Autodesk Inventor part; units mm, degrees
ref_plane "YZ Plane" through (0, 0, 0) normal (1, 0, 0) x (0, 1, 0)
ref_plane "XZ Plane" through (0, 0, 0) normal (0, 1, 0) x (-1, 0, 0)
ref_plane "XY Plane" through (0, 0, 0) normal (0, 0, 1) x (1, 0, 0)
sketch "Sketch1" plane through (0, 0, 0) normal (0, 1, 0) x (-1, 0, 0)
  line L0 (0, 0) -> (-215.9, 0)
  line L1 (-215.9, 0) -> (-215.9, -132.08)
  line L2 (-215.9, -132.08) -> (0, -132.08)
  line L3 (0, -132.08) -> (0, 0)
  circle A0 centre (-46.99, -129.008) radius 1.65
  circle A1 centre (-168.91, -129.008) radius 1.65
  circle A2 centre (-46.99, -3.072) radius 1.65
  circle A3 centre (-168.91, -3.072) radius 1.65
  circle A4 centre (-8, -50) radius 2.2
  circle A5 centre (-8, -100) radius 2.2
  circle A6 centre (-58, -50) radius 2.2
  circle A7 centre (-58, -100) radius 2.2
  circle A8 centre (-108, -50) radius 2.2
  circle A9 centre (-108, -100) radius 2.2
  circle A10 centre (-158, -50) radius 2.2
  circle A11 centre (-158, -100) radius 2.2
  circle A12 centre (-52.45, -72.08) radius 1.25
  circle A13 centre (-163.45, -72.08) radius 1.25
  circle A14 centre (-52.45, -33.08) radius 1.25
  circle A15 centre (-163.45, -33.08) radius 1.25
  dimension "d0" = 215.9
  dimension "d1" = 132.08
  dimension "d2" = 3.3
  dimension "d5" = 121.92
  dimension "d8" = 125.936
  dimension "d11" = 46.99
  dimension "d12" = 3.072
  dimension "d13" = 3.072
  dimension "d14" = 4.4
  dimension "d15" = 50
  dimension "d16" = 8
  dimension "d19" = 50
  dimension "d22" = 50
  dimension "d30" = 2.5
  dimension "d33" = 111
  dimension "d36" = 39
  dimension "d39" = 60
  dimension "d40" = 52.45
extrude "Extrusion1" add sketch "Sketch1" against normal blind 2.54
sketch "Sketch2" plane through (0, 0, 0) normal (0, 1, 0) x (1, 0, 0)
  line L0 (108.9107, 44.2653) -> (116.6369, 44.2653) construction
  line L1 (116.6369, 44.2653) -> (116.6369, 41.0888) construction
  line L2 (116.6369, 41.0888) -> (108.9107, 41.0888) construction
  line L3 (108.9107, 41.0888) -> (108.9107, 44.2653) construction
  point P0 (0, 0)
extrude "Extrusion2" [suppressed]
fillet "Fillet1" radius 5 4 edges at (0, -1.27, 0) (215.9, -1.27, 0) (215.9, -1.27, -132.08) (0, -1.27, -132.08)
sketch "Sketch3" plane through (0, 0, 0) normal (0, 1, 0) x (1, 0, 0)
  arc A0 (5, 132.08) -> (0, 127.08) centre (5, 127.08) ccw
  line L0 (0, 127.08) -> (0, 5)
  arc A1 (0, 5) -> (5, 0) centre (5, 5) ccw
  line L1 (5, 0) -> (210.9, 0)
  arc A2 (210.9, 0) -> (215.9, 5) centre (210.9, 5) ccw
  line L2 (215.9, 5) -> (215.9, 127.08)
  arc A3 (215.9, 127.08) -> (210.9, 132.08) centre (210.9, 127.08) ccw
  line L3 (210.9, 132.08) -> (5, 132.08)
  circle A4 centre (163.45, 33.08) radius 1.25
  circle A5 centre (163.45, 72.08) radius 1.25
  circle A6 centre (158, 100) radius 2.2
  circle A7 centre (108, 100) radius 2.2
  circle A8 centre (58, 100) radius 2.2
  circle A9 centre (58, 50) radius 2.2
  circle A10 centre (8, 100) radius 2.2
  circle A11 centre (8, 50) radius 2.2
  circle A12 centre (168.91, 3.072) radius 1.65
  circle A13 centre (46.99, 3.072) radius 1.65
  circle A14 centre (168.91, 129.008) radius 1.65
  circle A15 centre (46.99, 129.008) radius 1.65
  circle A16 centre (108, 50) radius 2.2
  circle A17 centre (158, 50) radius 2.2
  circle A18 centre (52.45, 72.08) radius 1.25
  circle A19 centre (52.45, 33.08) radius 1.25
  point P0 (0, 0)
equation "\"d40\" = -0.5 * d33 + 0.5 * d0"
properties part number "amplifier_tray"
Geometry check sheet. Reference: the model listing, model coordinates, mm. Round coordinates to 2 decimals unless told otherwise and drop trailing zeros. Order: outer loops, then holes, each group sorted by start corner. A loop starts at its lowest first (then second) coordinate and runs counter-clockwise, first axis right, second up. Notation, with made-up numbers: M 21,-38 L 68,-38 A26 ccw 68,-7 Z; hole C 49.5,-17.75 d11. An arc over 180 degrees is marked long. Answer as CSV lines item,"result".
1) Sectioned sample at A-A on x = 8. Record the cut outline in (y, z), and give its area (3 significant figures).
Entries:
outline,"M -2.54,-132.08 L 0,-132.08 L 0,-102.2 L -2.54,-102.2 Z; M -2.54,-97.8 L 0,-97.8 L 0,-52.2 L -2.54,-52.2 Z; M -2.54,-47.8 L 0,-47.8 L 0,0 L -2.54,0 Z"
area,"313 mm2"
2) Thickness scan on probe 1 along Z at (x, y) = (8, -1.1); probe 2 along Z at (x, y) = (46.99, -1.65). Record the ranges inside material, lowest first. Write a range as [from, to].
Entries:
probe 1,"[-132.08, -102.2], [-97.8, -52.2], [-47.8, 0]"
probe 2,"[-132.08, -130.66], [-127.36, -4.72], [-1.42, 0]"
3) Mould release check, pull along Z, two halves, no side actions. Record for faces 1 (the face through (1.43, -1.29, -130.58)), 2 (the face through (2, -1, -1)), 3 (the face through (6.817, -1.252, -98.145)), 4 (the face through (109.746, -1.252, -51.339)): +Z half, -Z half, draft (parallel to the pull), parting line (faces both ways), or undercut.
Entries:
face 1,"-Z half"
face 2,"+Z half"
face 3,"undercut"
face 4,"undercut"
